Print and shaded views of the part. All mm, measured from the part's lowest x, y and z. Round coordinates to 2 decimals unless told otherwise and drop trailing zeros. Loops run counter-clockwise (first coordinate to the right, second up) from the corner with the lowest first, then second, coordinate; pieces in that order, holes last. Notation, with made-up numbers: (-25.75, 29) - (33.25, 29) arc R14 cw to (33.25, 51) - close; hole circle Ø8 at (-31, 59). An arc over 180 degrees is marked (long way). Answer as a JSON object with one key per item and string values.
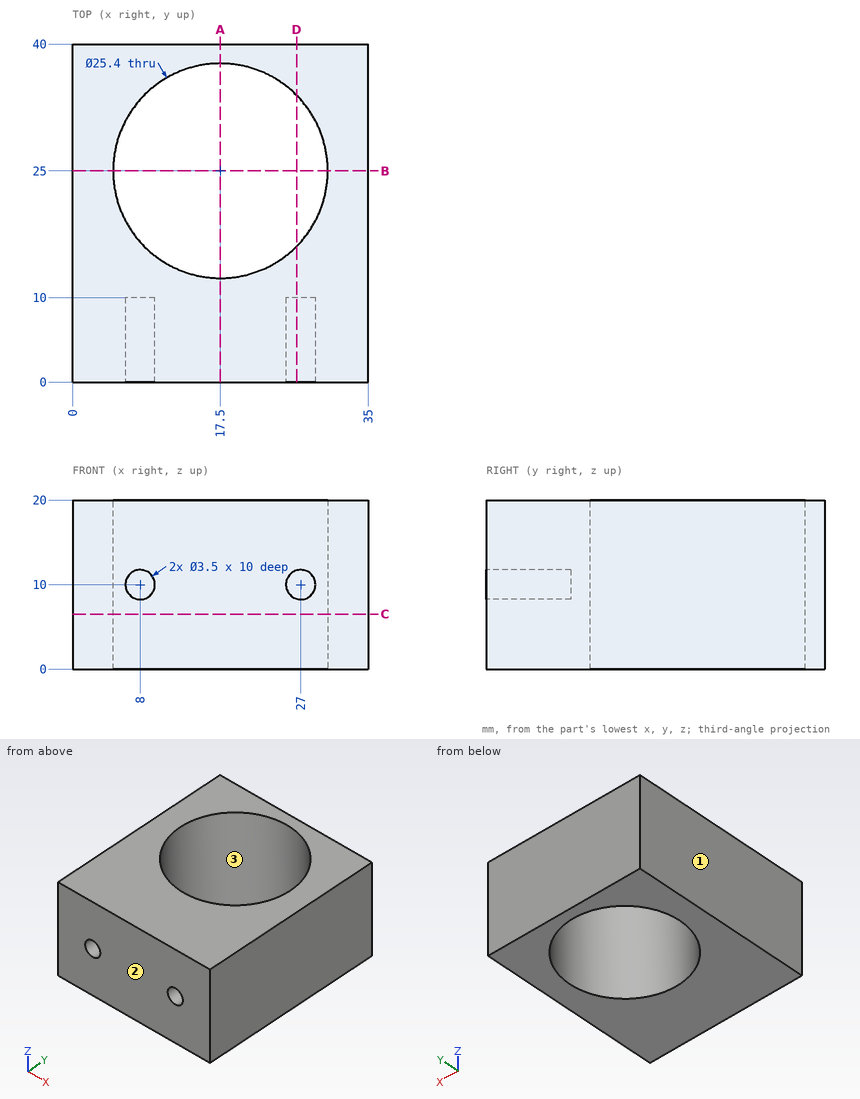
1) Probe probe 1 along Y at (x, z) = (17.5, 6.5); probe 2 along Z at (x, y) = (8, 5); probe 3 along X at (y, z) = (8, 9.25). List the from-to ranges inside material, lowest first.
Values follow:
{"probe 1": "0 to 12.3, 37.7 to 40", "probe 2": "0 to 8.25, 11.75 to 20", "probe 3": "0 to 6.42, 9.58 to 25.42, 28.58 to 35"}
2) Slice it at B-B on y = 25. List the corners of the cut face in (x, z), then the cut area to 3 significant figures.
Values follow:
{"outline": "(0, 0) - (4.8, 0) - (4.8, 20) - (0, 20) - close; (30.2, 0) - (35, 0) - (35, 20) - (30.2, 20) - close", "area": "192 mm²"}
3) Two-plate mould, pull along Y, no slides. Class the marked faces 1, 2 and 3: pulls with the +Y half, pulls with the -Y half, needs draft (parallel to the pull), parting line crosses it, or undercut.
Values follow:
{"face 1": "needs draft", "face 2": "pulls with the -Y half", "face 3": "undercut"}
4) Slice it at D-D on x = 26.5. List the corners of the cut face in (y, z), then the cut area to 3 significant figures.
Values follow:
{"outline": "(0, 0) - (16.04, 0) - (16.04, 20) - (0, 20) - (0, 11.68) - (10, 11.68) - (10, 8.32) - (0, 8.32) - close; (33.96, 0) - (40, 0) - (40, 20) - (33.96, 20) - close", "area": "408 mm²"}
5) Drop a flat-ended pin along its axis: P1, Ø1, axis at x = 27.5, z = 9, coming from the -Y side. Give the stop position or say it passes through.
Values follow:
{"P1": "y = 10"}
6) Slice it at A-A on x = 17.5. List the corners of the cut face in (y, z), then the cut area to 3 significant figures.
Values follow:
{"outline": "(0, 0) - (12.3, 0) - (12.3, 20) - (0, 20) - close; (37.7, 0) - (40, 0) - (40, 20) - (37.7, 20) - close", "area": "292 mm²"}
7) Slice it at C-C on z = 6.5. List the corners of the cut face in (x, y).
Values follow:
{"outline": "(0, 0) - (35, 0) - (35, 40) - (0, 40) - close; hole circle Ø25.4 at (17.5, 25)"}
